from build123d import *

# Parameters (mm, degrees)
F0_W     = 76.2
F0_H     = 76.2
F1_DEPTH = 3.175
F2_R     = 1
F3_DEPTH = 25.4
F4_W     = 57.15
F4_H     = 59.69
F5_DEPTH = 52
F6_R     = 1.0033
F7_DEPTH = 27.559


with BuildPart() as f1:
    # F0 (on Top) → F1 (new body)
    with BuildSketch(Plane.XY):
        Rectangle(F0_W, F0_H)
    extrude(amount=F1_DEPTH)

    # F2 (on face) → F3 (cut)
    with BuildSketch(Plane.XY.offset(3.175)):
        with Locations((-33.02, 33.02)):
            Circle(F2_R)
        with Locations((-33.02, -33.02)):
            Circle(F2_R)
        with Locations((33.02, 33.02)):
            Circle(F2_R)
        with Locations((33.02, -33.02)):
            Circle(F2_R)
    extrude(amount=-F3_DEPTH, mode=Mode.SUBTRACT)

    # F4 (on face) → F5 (join)
    with BuildSketch(Plane.XY.offset(3.175)):
        with Locations((0, 1.905)):
            Rectangle(F4_W, F4_H)
    extrude(amount=F5_DEPTH)

    # F6 (on face) → F7 (cut)
    with BuildSketch(Plane.XY.offset(55.175)):
        Polygon((10.16, -17.78), (10.16, 24.13), (-10.16, 24.13), (-10.16, -17.78), (-3.175, -17.78), (-3.175, -27.94), (3.175, -27.94), (3.175, -17.78), align=None)
        with Locations((-4.699, 27.686)):
            Circle(F6_R)
        with Locations((4.699, 27.686)):
            Circle(F6_R)
        with Locations((-4.699, -21.336)):
            Circle(F6_R)
        with Locations((4.699, -21.336)):
            Circle(F6_R)
    extrude(amount=-F7_DEPTH, mode=Mode.SUBTRACT)


solid = f1.part
Could you check a few things on this model? Use its own coordinates, in mm. A direction names the side the tool comes from. Coordinates: 2 decimals unless noted, no trailing zeros. Loops run counter-clockwise (first coordinate to the right, second up) from the corner with the lowest first, then second, coordinate; pieces in that order, holes last.
1. For P1, Ø3, axis at x = -3, y = -11.5, coming from the +Z side; P2, Ø4, axis at y = -17.5, z = 41.5, coming from the -X side (3 decimals); P3, Ø1.5, axis at y = 23.5, z = 46, coming from the +X side (3 decimals), each with a flat end and sliding along its axis, tell me the tip position at first contact or that it passes through.
2. For faces 4 (the face through (0, 31.75, 29)), 5 (the face through (3.175, -23, 42)), 6 (the face through (-4.916, -22.315, 41.588)), 7 (the face through (0, -27.94, 23)), which set-ups out of +Z, -Z, +X, -X, +Y, -Y let a thin tool reach every point of the face, with its end or its side?
3. We'd pull the mould along X, two halves only. Please class faces 1 (the face through (-38.1, -1, 2)), 2 (the face through (-10.16, 3, 42)), 3 (the face through (-34, 1, 3.175)): released by +X, released by -X, zero draft, split by the parting line, or undercut.
4. Imagine slicing it at A-A (y = 33.02). Please give me the cut outline in (x, z) (3 decimals).
5. I need wall thicknesses on L1, parallel to Y at x = -33.02, z = 0.65; L2, parallel to X at y = -27, z = 51.5 (3 decimals). Which ranges of each line are inside material? Lowest first, please.
6. Imagine slicing it at D-D (x = -14.5). Please give me the cut outline in (y, z) (3 decimals), and give its area (3 significant figures).
7. Imagine slicing it at C-C (y = -16.5). Please give me the cut outline in (x, z) (3 decimals), and give its area (3 significant figures).
Computed values:
1. P1: stops at z = 27.62
1. P2: stops at x = -28.575
1. P3: stops at x = 28.575
2. face 4: +Z, +X, -X, +Y
2. face 5: +Z, -Y
2. face 6: +Z
2. face 7: +Z, +X, -X, -Y
3. face 1: released by -X
3. face 2: undercut
3. face 3: zero draft
4. outline: (-38.1, 0) - (-34.02, 0) - (-34.02, 3.175) - (-38.1, 3.175) - close; (-32.02, 0) - (32.02, 0) - (32.02, 3.175) - (-32.02, 3.175) - close; (34.02, 0) - (38.1, 0) - (38.1, 3.175) - (34.02, 3.175) - close
5. L1: y = -38.1 to -34.02, -32.02 to 32.02, 34.02 to 38.1
5. L2: x = -28.575 to -3.175, 3.175 to 28.575
6. outline: (-38.1, 0) - (38.1, 0) - (38.1, 3.175) - (31.75, 3.175) - (31.75, 55.175) - (-27.94, 55.175) - (-27.94, 3.175) - (-38.1, 3.175) - close
6. area: 3,350 mm2
7. outline: (-38.1, 0) - (38.1, 0) - (38.1, 3.175) - (28.575, 3.175) - (28.575, 55.175) - (10.16, 55.175) - (10.16, 27.616) - (-10.16, 27.616) - (-10.16, 55.175) - (-28.575, 55.175) - (-28.575, 3.175) - (-38.1, 3.175) - close
7. area: 2,650 mm2
